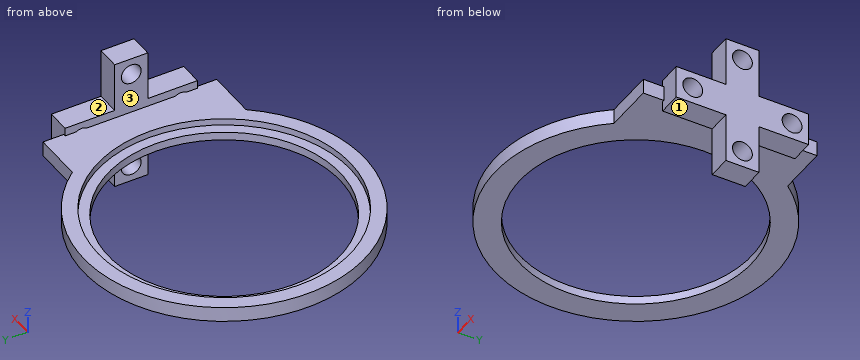
```python
from build123d import *

# Parameters (mm, degrees)
F0_R     = 42.4
F0_R_2   = 35
F1_DEPTH = 2.5
F2_R     = 42.4
F2_R_2   = 38.1
F3_DEPTH = 2
F7_DEPTH = 4.5
F8_START = 3.2
F5_R     = 3
F8_DEPTH = 7


with BuildPart() as f1:
    # F0 (on Top) → F1 (new body)
    with BuildSketch(Plane.XY):
        Circle(F0_R)
        Circle(F0_R_2, mode=Mode.SUBTRACT)
    extrude(amount=F1_DEPTH)

    # F2 (on face) → F3 (join)
    with BuildSketch(Plane.XY.offset(2.5)):
        Circle(F2_R)
        Circle(F2_R_2, mode=Mode.SUBTRACT)
    extrude(amount=F3_DEPTH)

    # F6 (on face) → F7 (join)
    with BuildSketch(Plane.XY.offset(4.5)):
        with BuildLine():
            Line((48.2971094842, -26.25), (48.2971094842, 26.25))
            Line((48.2971094842, 26.25), (33.2971094842, 26.25))
            ThreePointArc((33.2971094842, 26.25), (42.4, 0), (33.2971094842, -26.25))
            Line((33.2971094842, -26.25), (48.2971094842, -26.25))
        make_face()
    extrude(amount=-F7_DEPTH)

    # F5 (on offset) → F8 (join)
    with BuildSketch(Plane.YZ.offset(44.38663).offset(F8_START)):
        Polygon((20, -3), (20, 7), (5, 7), (5, 22), (-5, 22), (-5, 7), (-20, 7), (-20, -3), (-5, -3), (-5, -18), (5, -18), (5, -3), align=None)
        with Locations((0, -13)):
            Circle(F5_R, mode=Mode.SUBTRACT)
        with Locations((-15, 2)):
            Circle(F5_R, mode=Mode.SUBTRACT)
        with Locations((15, 2)):
            Circle(F5_R, mode=Mode.SUBTRACT)
        with Locations((0, 17)):
            Circle(F5_R, mode=Mode.SUBTRACT)
    extrude(amount=F8_DEPTH)


solid = f1.part
```
Build history of the part. All positions in model axes, mm. Face numbers are marked on the shaded views. A direction names the side the tool comes from. Round coordinates to 2 decimals unless told otherwise and drop trailing zeros. Write each loop counter-clockwise with the first axis right and the second up, starting at its lowest first coordinate (ties: lowest second). Pieces come first, ordered by that corner, then holes. Notation, with made-up numbers: (-15, -24) -> (-2, -24) arc R18 ccw to (-2, -9) -> close; hole circle Ø4 at (72.5, -29). An arc over 180 degrees is marked (long way). Put each result on its own line as item: value.
Item 1: Tool access for the marked faces 1, 2 and 3: list every direction of +Z, -Z, +X, -X, +Y, -Y with a clear straight run to the whole face (end or side of a thin tool).
Here are the results:
face 1: -Z, +X, -X, -Y
face 2: +Z, +X, -X, +Y
face 3: +Z, -X, +Y, -Y
Item 2: Slice it at B-B, the plane z = 17. Give the cut face in (x, y), plus the area to 3 significant figures.
Here are the results:
outline: (47.59, -5) -> (54.59, -5) -> (54.59, -3) -> (47.59, -3) -> close; (47.59, 3) -> (54.59, 3) -> (54.59, 5) -> (47.59, 5) -> close
area: 28.0 mm^2
Item 3: Slice it at C-C, the plane y = 0. Give the cut face in (x, z), plus the area to 3 significant figures.
Here are the results:
outline: (-42.4, 0) -> (-35, 0) -> (-35, 2.5) -> (-38.1, 2.5) -> (-38.1, 4.5) -> (-42.4, 4.5) -> close; (35, 0) -> (47.59, 0) -> (47.59, -10) -> (54.59, -10) -> (54.59, 14) -> (47.59, 14) -> (47.59, 4.5) -> (38.1, 4.5) -> (38.1, 2.5) -> (35, 2.5) -> close; (47.59, -18) -> (54.59, -18) -> (54.59, -16) -> (47.59, -16) -> close; (47.59, 20) -> (54.59, 20) -> (54.59, 22) -> (47.59, 22) -> close
area: 274 mm^2
Item 4: Flat gauge pins, fed straight in: P1, Ø2, axis at x = 50.5, y = -11.5, coming from the +Z side; P2, Ø3.5, axis at x = 51, y = 9, coming from the -Z side; P3, Ø5, axis at x = 27, z = 0.5, coming from the -Y side. Where does each tip first touch, or does it go through?
Here are the results:
P1: stops at z = 7
P2: stops at z = -3
P3: stops at y = -34.61
Item 5: Slice it at A-A, the plane x = 0. Give the cut face in (y, z).
Here are the results:
outline: (-42.4, 0) -> (-35, 0) -> (-35, 2.5) -> (-38.1, 2.5) -> (-38.1, 4.5) -> (-42.4, 4.5) -> close; (35, 0) -> (42.4, 0) -> (42.4, 4.5) -> (38.1, 4.5) -> (38.1, 2.5) -> (35, 2.5) -> close
Item 6: Wall check: probe 1 along Y at (x, z) = (52, 2); probe 2 along Z at (x, y) = (52, -15); probe 3 along Y at (x, z) = (0, 3). Give the ranges that are in metal, low to high. Write a range as from..to.
Here are the results:
probe 1: y = -20..-18, -12..12, 18..20
probe 2: z = -3..-1, 5..7
probe 3: y = -42.4..-38.1, 38.1..42.4
Item 7: Slice it at D-D, the plane y = -15. Give the cut face in (x, z), plus the area to 3 significant figures.
Here are the results:
outline: (-39.66, 0) -> (-31.62, 0) -> (-31.62, 2.5) -> (-35.02, 2.5) -> (-35.02, 4.5) -> (-39.66, 4.5) -> close; (31.62, 0) -> (48.3, 0) -> (48.3, 4.5) -> (35.02, 4.5) -> (35.02, 2.5) -> (31.62, 2.5) -> close; (47.59, -3) -> (54.59, -3) -> (54.59, -1) -> (47.59, -1) -> close; (47.59, 5) -> (54.59, 5) -> (54.59, 7) -> (47.59, 7) -> close
area: 126 mm^2
